The drawing under review shows one solid part. Ordinate dimensions are in mm from its lowest x, y, z. A direction names the side the tool comes from. Give positions to 0.01 mm unless a question says otherwise; leave off trailing zeros. Write each loop counter-clockwise with the first axis right and the second up, starting at its lowest first coordinate (ties: lowest second). Pieces come first, ordered by that corner, then holes. Notation, with made-up numbers: (66, 24) -> (76, 24) arc R8 ccw to (76, 32) -> close; hole circle Ø8 at (48, -13.5). An arc over 180 degrees is marked (long way). Write item = value, one per line.
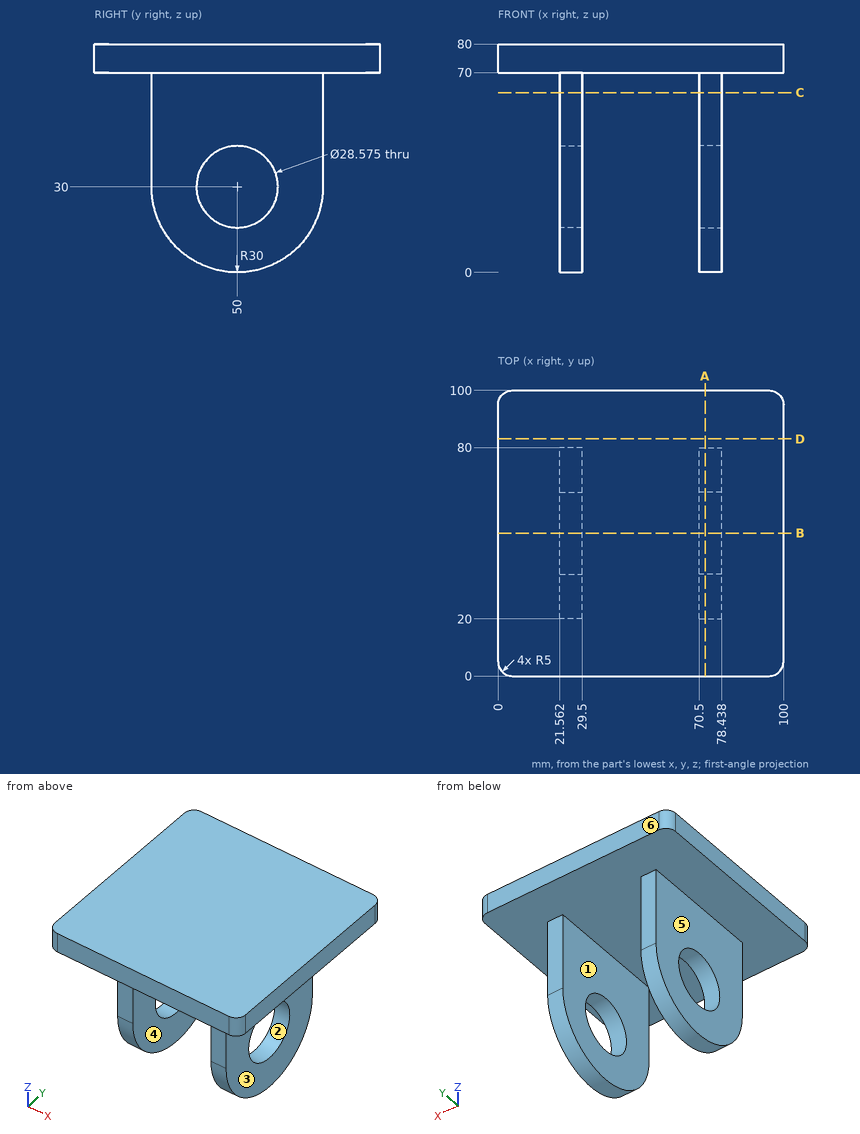
(1) For pin 1 (18 mm diameter, centred on y = 56, z = 29.5, fed in from -X); pin 2 (2.5 mm diameter, centred on x = 24.5, z = 45.5, fed in from -Y); pin 3 (10 mm diameter, centred on x = 36.5, z = 62.5, fed in from -Y); pin 4 (10 mm diameter, centred on x = 32.5, y = 50.5, fed in from -Z), all flat-tipped, find the tip position at first contact; note any pin that passes through.
Answers below:
pin_1 = 21.56
pin_2 = 20
pin_3 = through
pin_4 = 0
(2) Tool access review of the marked faces 4, 5 and 6: name each direction out of +Z, -Z, +X, -X, +Y, -Y from which nothing blocks a thin tool from reaching the whole face with its end or side.
Answers below:
face_4 = -Z, +Y, -Y
face_5 = -Z, -X, +Y, -Y
face_6 = +Z, -Z, +X, -X, +Y
(3) Take a section at C-C (z = 63). Write out the cut boundary in (x, y).
Answers below:
outline = (21.56, 20) -> (29.5, 20) -> (29.5, 80) -> (21.56, 80) -> close; (70.5, 20) -> (78.44, 20) -> (78.44, 80) -> (70.5, 80) -> close
(4) To check wall thickness, follow probe 1 along X at (y, z) = (26, 57); probe 2 along Y at (x, z) = (75, 30); probe 3 along Z at (x, y) = (62, 71). State the ranges of each line that lie inside material, in increasing order.
Answers below:
probe_1 = 21.56 to 29.5, 70.5 to 78.44
probe_2 = 20 to 35.71, 64.29 to 80
probe_3 = 70 to 80
(5) Take a section at A-A (x = 72.5). Write out the cut boundary in (y, z) (1 decimal).
Answers below:
outline = (0, 70) -> (20, 70) -> (20, 30) arc R30 ccw to (80, 30) -> (80, 70) -> (100, 70) -> (100, 80) -> (0, 80) -> close; hole circle Ø28.6 at (50, 30)
(6) The part is to be moulded in two halves that separate along X. For the marked faces 1, 2 and 3, say which applies: released by +X, released by -X, zero draft, split by the parting line, or undercut.
Answers below:
face_1 = undercut
face_2 = zero draft
face_3 = released by +X
(7) Take a section at B-B (y = 50). Write out the cut boundary in (x, z).
Answers below:
outline = (0, 70) -> (21.56, 70) -> (21.56, 44.29) -> (29.5, 44.29) -> (29.5, 70) -> (70.5, 70) -> (70.5, 44.29) -> (78.44, 44.29) -> (78.44, 70) -> (100, 70) -> (100, 80) -> (0, 80) -> close; (21.56, 0) -> (29.5, 0) -> (29.5, 15.71) -> (21.56, 15.71) -> close; (70.5, 0) -> (78.44, 0) -> (78.44, 15.71) -> (70.5, 15.71) -> close
(8) Take a section at D-D (y = 83). Write out the cut boundary in (x, z).
Answers below:
outline = (0, 70) -> (100, 70) -> (100, 80) -> (0, 80) -> close
